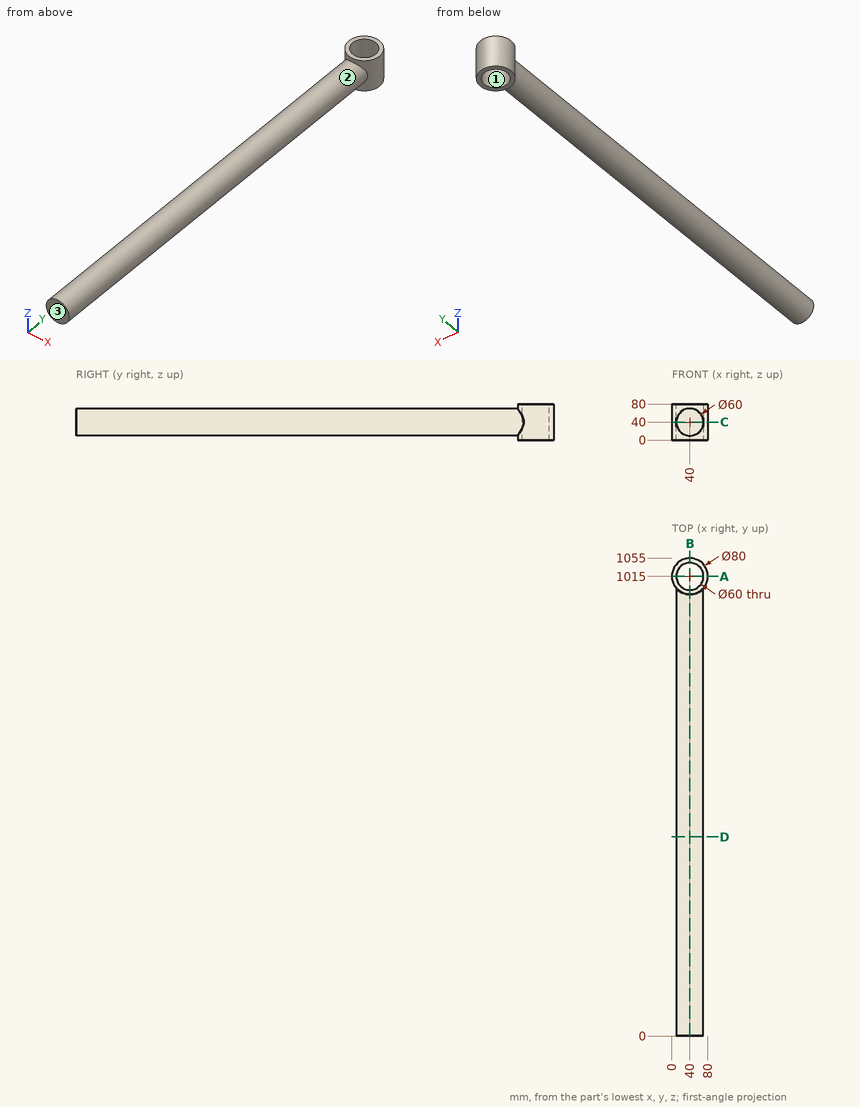
Here's the drawing with two shaded views (mm, measured from the low corner). I have some questions. Round coordinates to 2 decimals unless told otherwise and drop trailing zeros. Order: outer loops, then holes, each group sorted by start corner. A loop starts at its lowest first (then second) coordinate and runs counter-clockwise, first axis right, second up. Notation, with made-up numbers: M 67.5,-31 L 110.5,-31 A14 cw 110.5,-5 Z; hole C -26.5,4 d1. An arc over 180 degrees is marked long. Answer in a Markdown table with one row per item.
Item 1: Thinking about a two-plate mould opening in X: for the marked faces 1, 2 and 3, which applies, +X half, -X half, draft (parallel to the pull), parting line (faces both ways), or undercut?
A:
| item | result |
|---|---|
| face 1 | undercut |
| face 2 | parting line |
| face 3 | draft |
Item 2: I'm going to push flat-ended pins straight in: pin 1 (10 mm diameter, centred on x = 49.5, z = 26.5, fed in from +Y); pin 2 (6 mm diameter, centred on y = 467.5, z = 62, fed in from +X); pin 3 (8 mm diameter, centred on x = 33.5, z = 37, fed in from +Y). Where does each tip first touch, or does it pass through?
A:
| item | result |
|---|---|
| pin 1 | stops at y = 1054.75 |
| pin 2 | stops at x = 63.22 |
| pin 3 | stops at y = 1054.92 |
Item 3: Imagine slicing it at C-C, the plane z = 40. Write out the boundary of the cut face in (x, y), and give its area (3 significant figures).
A:
| item | result |
|---|---|
| outline | M 10,0 L 70,0 L 70,988.54 A40 ccw long 10,988.54 Z; hole C 40,1015 d60 |
| area | 60,900 mm2 |
Item 4: Imagine slicing it at A-A, the plane y = 1015. Write out the boundary of the cut face in (x, z), and give its area (3 significant figures).
A:
| item | result |
|---|---|
| outline | M 0,0 L 10,0 L 10,80 L 0,80 Z; M 70,0 L 80,0 L 80,80 L 70,80 Z |
| area | 1,600 mm2 |
Item 5: Imagine slicing it at B-B, the plane x = 40. Write out the boundary of the cut face in (y, z).
A:
| item | result |
|---|---|
| outline | M 0,10 L 975,10 L 975,0 L 985,0 L 985,80 L 975,80 L 975,70 L 0,70 Z; M 1045,0 L 1055,0 L 1055,80 L 1045,80 Z |
Item 6: Imagine slicing it at D-D, the plane y = 439.5. Write out the boundary of the cut face in (x, z).
A:
| item | result |
|---|---|
| outline | C 40,40 d60 |
Item 7: If I drill on L1, parallel to Y at x = 40, z = 29; L2, parallel to X at y = 416, z = 43.5; L3, parallel to Y at x = 29, z = 71, over which ranges is the centre line in solid material (lowest first)? Write a range as from..to.
A:
| item | result |
|---|---|
| L1 | y = 0..985, 1045..1055 |
| L2 | x = 10.2..69.8 |
| L3 | y = 976.54..987.09, 1042.91..1053.46 |
